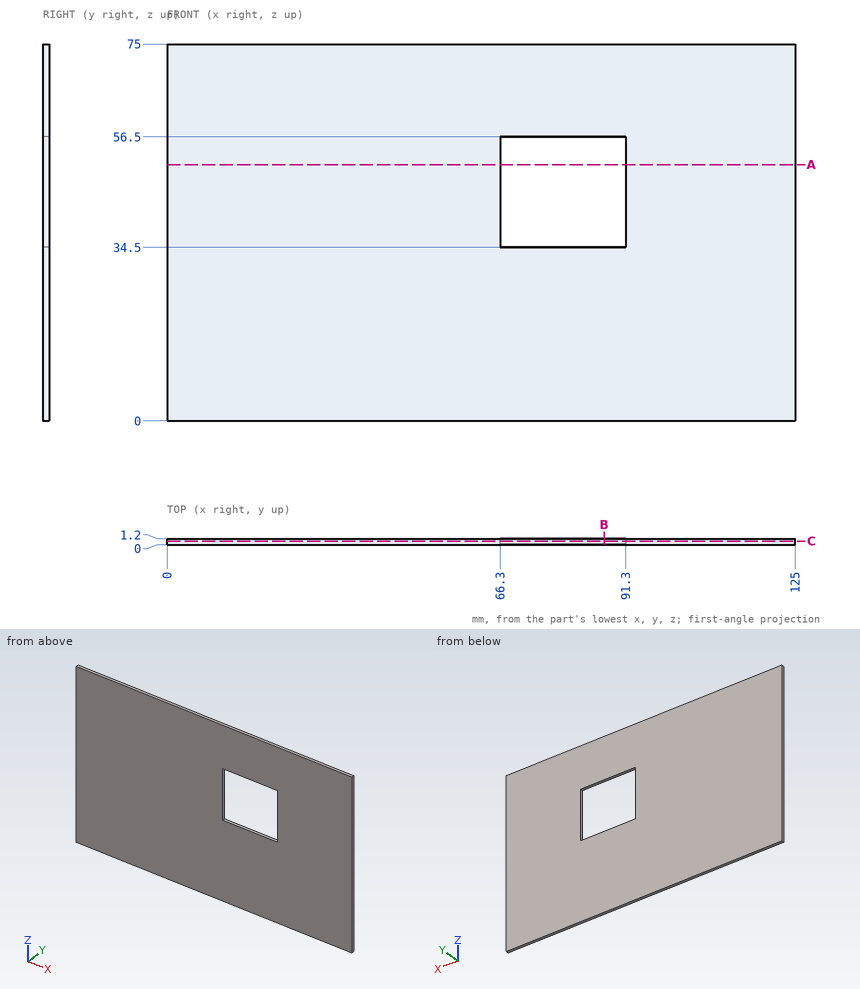
Part print with two shaded views. Sizes in mm from the minimum x, y, z corner. Give positions to 0.01 mm unless a question says otherwise; leave off trailing zeros. Order: outer loops, then holes, each group sorted by start corner. A loop starts at its lowest first (then second) coordinate and runs counter-clockwise, first axis right, second up.
1) Saw through at B-B, the plane x = 87. Write the cut outline in (y, z).
2) Saw through at C-C, the plane y = 0.75. Write the cut outline in (x, z), then the cut area to 4 significant figures.
3) Wall check: probe 1 along Z at (x, y) = (83, 0.55); probe 2 along X at (y, z) = (0.6, 48.5). Give the ranges that are in metal, low to high.
4) Saw through at A-A, the plane z = 51. Write the cut outline in (x, y).
Computed:
1. outline: (0, 0) - (1.2, 0) - (1.2, 34.5) - (0, 34.5) - close; (0, 56.5) - (1.2, 56.5) - (1.2, 75) - (0, 75) - close
2. outline: (0, 0) - (125, 0) - (125, 75) - (0, 75) - close; hole (66.3, 34.5) - (91.3, 34.5) - (91.3, 56.5) - (66.3, 56.5) - close
2. area: 8,825 mm2
3. probe 1: z = 0 to 34.5, 56.5 to 75
3. probe 2: x = 0 to 66.3, 91.3 to 125
4. outline: (0, 0) - (66.3, 0) - (66.3, 1.2) - (0, 1.2) - close; (91.3, 0) - (125, 0) - (125, 1.2) - (91.3, 1.2) - close
